Source: CAD feature listing. Evaluate the final solid. Frame: model axes, mm. Face numbers are marked on the shaded views. A direction names the side the tool comes from. Coordinates: 2 decimals unless noted, no trailing zeros. Loops run counter-clockwise (first coordinate to the right, second up) from the corner with the lowest first, then second, coordinate; pieces in that order, holes last.
Item 1: Reachability of the marked faces 4 and 5 from +Z, -Z, +X, -X, +Y, -Y: full face, straight path, thin tool, end or side. Return the list, or none.
Item 2: Pin query (flat end, axial travel): pin 1 Ø3.5 at (x, z) = (1, 7.5) entering from +Y; pin 2 Ø1 at (x, y) = (-15, -12) entering from -Z. Return the tip coordinate at first contact, or that it passes through.
Item 3: Section query B-B, the plane z = 6.75. Return the cut outline in (x, y).
Item 4: Section query C-C, the plane x = 5. Return the cut outline in (y, z).
Item 5: Pull-direction query (X, two-part tool) for the marked faces 1, 2 and 3; classes: +X half, -X half, draft (parallel to the pull), parting line (faces both ways), or undercut.
Item 6: Line query: probe 1 along X at (y, z) = (29, 4.25); probe 2 along Y at (x, z) = (5, 6.5). Output: solid intervals per line, ascending.
Item 7: Section query A-A, the plane y = 23. Return the cut outline in (x, z), then the cut area to 3 significant figures.
```python
from build123d import *

# Parameters (mm, degrees)
SZKIC1_W                    = 40
SZKIC1_H                    = 70
DODANIE_WYCI_GNI_CIE1_DEPTH = 12
SZKIC2_W                    = 20
SZKIC2_H                    = 18
WYTNIJ_WYCI_GNI_CIE1_DEPTH  = 43.05948169


with BuildPart() as part:
    # Szkic1 → Dodanie-wyciągnięcie1 (new body)
    with BuildSketch(Plane.XY):
        Rectangle(SZKIC1_W, SZKIC1_H)
    extrude(amount=DODANIE_WYCI_GNI_CIE1_DEPTH)

    # Szkic2 → Wytnij-wyciągnięcie1 (cut, through all)
    with BuildSketch(Plane.XY.offset(12)):
        with Locations((0, 26)):
            Rectangle(SZKIC2_W, SZKIC2_H)
    extrude(amount=-WYTNIJ_WYCI_GNI_CIE1_DEPTH, mode=Mode.SUBTRACT)


solid = part.part
```
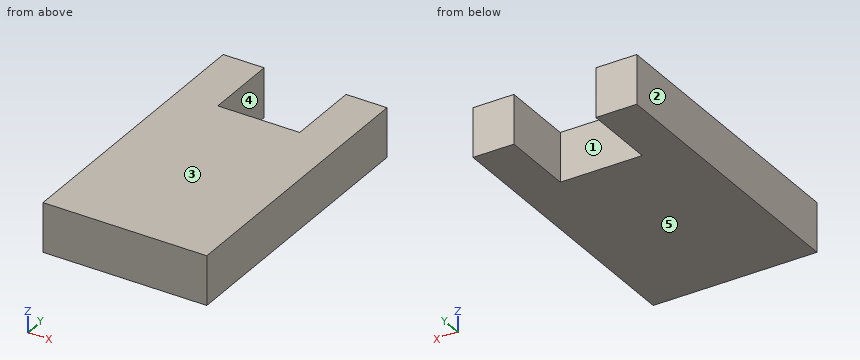
Verdict:
1. face 4: +Z, -Z, +Y
1. face 5: -Z, +X, -X, +Y, -Y
2. pin 1: stops at y = 17
2. pin 2: stops at z = 0
3. outline: (-20, -35) - (20, -35) - (20, 35) - (10, 35) - (10, 17) - (-10, 17) - (-10, 35) - (-20, 35) - close
4. outline: (-35, 0) - (17, 0) - (17, 12) - (-35, 12) - close
5. face 1: undercut
5. face 2: -X half
5. face 3: draft
6. probe 1: x = -20 to -10, 10 to 20
6. probe 2: y = -35 to 17
7. outline: (-20, 0) - (-10, 0) - (-10, 12) - (-20, 12) - close; (10, 0) - (20, 0) - (20, 12) - (10, 12) - close
7. area: 240 mm2
